Geometry check sheet. Reference: drawing and pictorial views, mm from the part's lowest x, y, z. Give positions to 0.01 mm unless a question says otherwise; leave off trailing zeros. Order: outer loops, then holes, each group sorted by start corner. A loop starts at its lowest first (then second) coordinate and runs counter-clockwise, first axis right, second up. Notation, with made-up numbers: M 83,54 L 139,54 A22 cw 139,91 Z; hole C 89,82 d5. An arc over 180 degrees is marked long. Use CSV: the item, a comma, the result in double quotes. Start each with the question number.
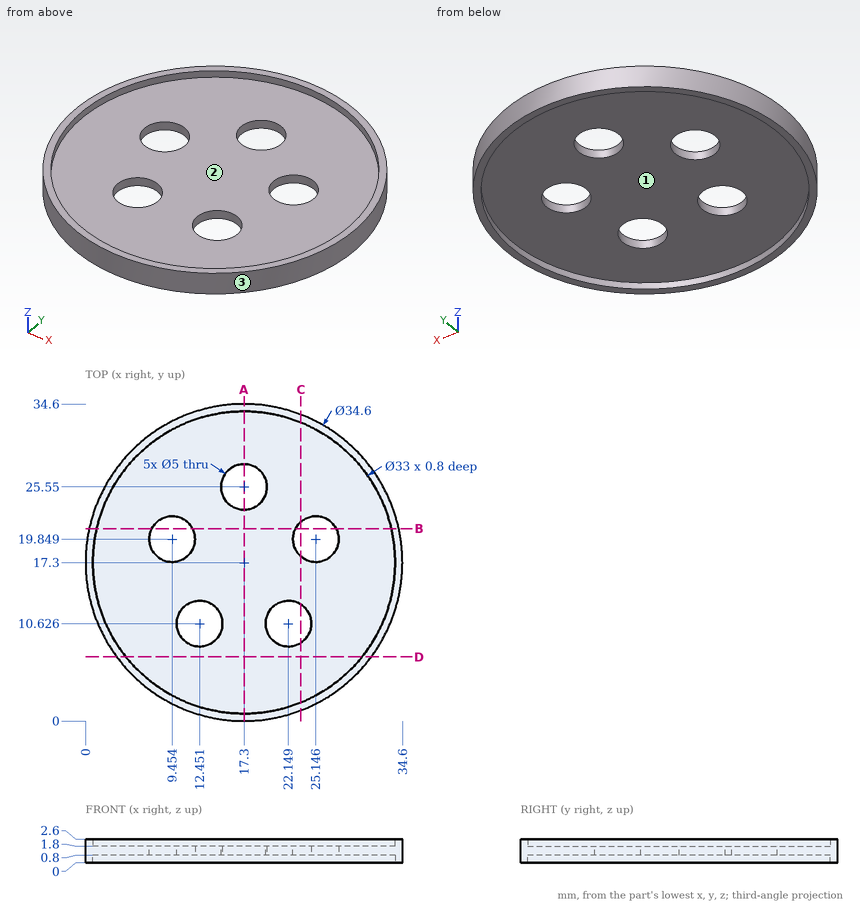
(1) Sectioned sample at C-C on x = 23.5. Record the cut outline in (y, z).
(2) Sectioned sample at D-D on y = 7. Record the cut outline in (x, z).
(3) Thickness scan on line 1 (Y direction, x = 11, z = 1.75) (1 decimal); line 2 (Y direction, x = 17.3, z = 2.1); line 3 (Z direction, x = 10.5, y = 15.5). Record the ranges inside material, lowest first.
(4) Sectioned sample at B-B on y = 21. Record the cut outline in (x, z) (1 decimal).
(5) Draft check along X on the marked faces 1, 2 and 3. Enter one of: +X half, -X half, draft (parallel to the pull), parting line (faces both ways), or undercut.
(6) Sectioned sample at A-A on x = 17.3. Record the cut outline in (y, z).
(7) Go/stop test with flat-tipped pins: P1, Ø4, axis at x = 12.45, y = 10.63, coming from the -Z side; P2, Ø8, axis at x = 9.45, y = 19.85, coming from the -Z side; P3, Ø6, axis at x = 22.15, y = 10.63, coming from the +Z side; P4, Ø1, axis at x = 14.5, z = 1.5, coming from the +Y side. Record where each tip stops, or that it passes through.
Responses:
1,outline,"M 1.15,0 L 2.01,0 L 2.01,0.8 L 8.52,0.8 L 8.52,1.8 L 2.01,1.8 L 2.01,2.6 L 1.15,2.6 Z; M 12.73,0.8 L 17.97,0.8 L 17.97,1.8 L 12.73,1.8 Z; M 21.73,0.8 L 32.59,0.8 L 32.59,0 L 33.45,0 L 33.45,2.6 L 32.59,2.6 L 32.59,1.8 L 21.73,1.8 Z"
2,outline,"M 3.4,0 L 4.41,0 L 4.41,0.8 L 30.19,0.8 L 30.19,0 L 31.2,0 L 31.2,2.6 L 30.19,2.6 L 30.19,1.8 L 4.41,1.8 L 4.41,2.6 L 3.4,2.6 Z"
3,line 1,"1.2 to 8.6, 12.7 to 17.9, 21.8 to 33.4"
3,line 2,"0 to 0.8, 33.8 to 34.6"
3,line 3,"0.8 to 1.8"
4,outline,"M 0.4,0 L 1.2,0 L 1.2,0.8 L 7.2,0.8 L 7.2,1.8 L 1.2,1.8 L 1.2,2.6 L 0.4,2.6 Z; M 11.7,0.8 L 22.9,0.8 L 22.9,1.8 L 11.7,1.8 Z; M 27.4,0.8 L 33.4,0.8 L 33.4,0 L 34.2,0 L 34.2,2.6 L 33.4,2.6 L 33.4,1.8 L 27.4,1.8 Z"
5,face 1,"undercut"
5,face 2,"undercut"
5,face 3,"parting line"
6,outline,"M 0,0 L 0.8,0 L 0.8,0.8 L 23.05,0.8 L 23.05,1.8 L 0.8,1.8 L 0.8,2.6 L 0,2.6 Z; M 28.05,0.8 L 33.8,0.8 L 33.8,0 L 34.6,0 L 34.6,2.6 L 33.8,2.6 L 33.8,1.8 L 28.05,1.8 Z"
7,P1,"through"
7,P2,"z = 0.8"
7,P3,"z = 1.8"
7,P4,"y = 34.45"
